Could you check a few things on this model? Use its own coordinates, in mm. Face numbers are marked on the shaded views. A direction names the side the tool comes from. Give positions to 0.01 mm unless a question says otherwise; leave off trailing zeros. Order: outer loops, then holes, each group sorted by start corner. A loop starts at its lowest first (then second) coordinate and runs counter-clockwise, first axis right, second up. Notation, with made-up numbers: (67.5, 76) -> (83.5, 76) arc R30 ccw to (83.5, 98) -> close; hole circle Ø4 at (-5, -13). An arc over 180 degrees is marked (long way). Write each question's results on one line, items separated by ' | '.
```python
from build123d import *

# Parameters (mm, degrees)
BOSS_EXTRU_1_DEPTH                                   = 15
ESQUISSE2_W                                          = 10
ESQUISSE2_H                                          = 25
ESQUISSE2_H_2                                        = 5
BOSS_EXTRU_2_DEPTH                                   = 6
D_GAGEMENT_M1_21_D                                   = 1.4
CHAMBRAGE_POUR_T_TE_CYLINDRIQUE_FENDUE_M_D           = 3.4
CHAMBRAGE_POUR_T_TE_CYLINDRIQUE_FENDUE_M_CBORE_D     = 6.5
CHAMBRAGE_POUR_T_TE_CYLINDRIQUE_FENDUE_M_CBORE_DEPTH = 2
CONG_1_R                                             = 10


with BuildPart() as part:
    # Esquisse1 → Boss.-Extru.1 (new body)
    with BuildSketch(Plane.XY):
        Polygon((0, 0), (-20, 0), (-20, 6), (-13, 6), (-13, 76), (13, 76), (13, 6), (20, 6), (20, 0), align=None)
    extrude(amount=BOSS_EXTRU_1_DEPTH)

    # Esquisse2 → Boss.-Extru.2 (add)
    with BuildSketch(Plane.XZ):
        with Locations((15, 27.5)):
            Rectangle(ESQUISSE2_W, ESQUISSE2_H)
        with Locations((-15, 17.5)):
            Rectangle(ESQUISSE2_W, ESQUISSE2_H_2)
    extrude(amount=-BOSS_EXTRU_2_DEPTH)

    # Dégagement M1.21 (through all)
    with Locations(Plane.XY.offset(15)):
        with Locations((0, 62), (0, 40)):
            Hole(D_GAGEMENT_M1_21_D / 2)

    # Chambrage pour tête cylindrique fendue M31 (through all)
    with Locations(Plane(origin=(0, 6, 0), x_dir=(1, 0, 0), z_dir=(0, 1, 0))):
        with Locations((-16.5, -5), (16.5, -5), (16.5, -35)):
            CounterBoreHole(CHAMBRAGE_POUR_T_TE_CYLINDRIQUE_FENDUE_M_D / 2, CHAMBRAGE_POUR_T_TE_CYLINDRIQUE_FENDUE_M_CBORE_D / 2, CHAMBRAGE_POUR_T_TE_CYLINDRIQUE_FENDUE_M_CBORE_DEPTH)

    # Congé1
    cong_1_edges = [part.edges().sort_by_distance(p)[0] for p in [
        (-13, 76, 7.5),
        (13, 76, 7.5),
    ]]
    fillet(cong_1_edges, radius=CONG_1_R)


solid = part.part
```
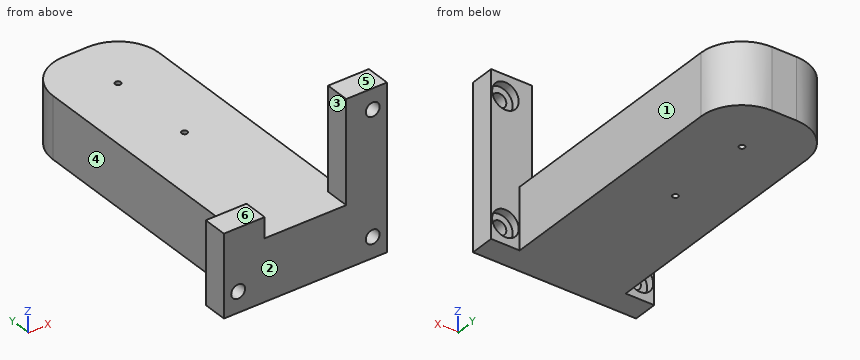
Q1. Suppose I cut it at B-B on x = 16.5. Please give me the cut outline in (y, z).
Here are the results:
outline: (0, 0) -> (6, 0) -> (6, 1.75) -> (4, 1.75) -> (4, 3.3) -> (0, 3.3) -> close; (0, 6.7) -> (4, 6.7) -> (4, 8.25) -> (6, 8.25) -> (6, 31.75) -> (4, 31.75) -> (4, 33.3) -> (0, 33.3) -> close; (0, 36.7) -> (4, 36.7) -> (4, 38.25) -> (6, 38.25) -> (6, 40) -> (0, 40) -> close
Q2. Suppose I cut it at A-A on z = 5. Please give me the cut outline in (x, y), and give its area (3 significant figures).
Here are the results:
outline: (-20, 0) -> (-18.2, 0) -> (-18.2, 4) -> (-19.75, 4) -> (-19.75, 6) -> (-20, 6) -> close; (-14.8, 0) -> (14.8, 0) -> (14.8, 4) -> (13.25, 4) -> (13.25, 6) -> (13, 6) -> (13, 66) arc R10 ccw to (3, 76) -> (-3, 76) arc R10 ccw to (-13, 66) -> (-13, 6) -> (-13.25, 6) -> (-13.25, 4) -> (-14.8, 4) -> close; (18.2, 0) -> (20, 0) -> (20, 6) -> (19.75, 6) -> (19.75, 4) -> (18.2, 4) -> close; hole circle Ø1.4 at (0, 40); hole circle Ø1.4 at (0, 62) | area: 1,960 mm²
Q3. Suppose I cut it at C-C on z = 35. Please give me the cut outline in (x, y).
Here are the results:
outline: (10, 0) -> (14.8, 0) -> (14.8, 4) -> (13.25, 4) -> (13.25, 6) -> (10, 6) -> close; (18.2, 0) -> (20, 0) -> (20, 6) -> (19.75, 6) -> (19.75, 4) -> (18.2, 4) -> close
Q4. I need wall thicknesses on line 1 along X through (y, z) = (1, 5); line 2 along Z through (x, y) = (16.5, 2.05); line 3 along Y through (x, z) = (0, 10.5). Which ranges of each line are inside material? Lowest first, please.
Here are the results:
line 1: x = -20 to -18.2, -14.8 to 14.8, 18.2 to 20 | line 2: z = 0 to 3.3, 6.7 to 33.3, 36.7 to 40 | line 3: y = 0 to 39.3, 40.7 to 61.3, 62.7 to 76
Q5. I'm going to push flat-ended pins straight in: pin 1 Ø8 at (y, z) = (17, 10.5) entering from +X; pin 2 Ø1.8 at (x, y) = (0, 62) entering from -Z; pin 3 Ø5 at (x, z) = (-17, 4.5) entering from +Y; pin 4 Ø10.5 at (x, z) = (-16.5, 5) entering from +Y. Where does each tip first touch, or does it pass through?
Here are the results:
pin 1: stops at x = 13 | pin 2: stops at z = 0 | pin 3: stops at y = 4 | pin 4: stops at y = 71.65
Q6. Suppose I cut it at D-D on x = -16. Please give me the cut outline in (y, z), and give its area (3 significant figures).
Here are the results:
outline: (0, 0) -> (6, 0) -> (6, 1.79) -> (4, 1.79) -> (4, 3.38) -> (0, 3.38) -> close; (0, 6.62) -> (4, 6.62) -> (4, 8.21) -> (6, 8.21) -> (6, 20) -> (0, 20) -> close | area: 94.2 mm²
Q7. For the marked faces 5 and 6, which set-ups out of +Z, -Z, +X, -X, +Y, -Y let a thin tool reach every point of the face, with its end or its side?
Here are the results:
face 5: +Z, +X, -X, +Y, -Y | face 6: +Z, -X, +Y, -Y
Q8. Thinking about a two-plate mould opening in X: for the marked faces 1, 2, 3 and 4, which applies, +X half, -X half, draft (parallel to the pull), parting line (faces both ways), or undercut?
Here are the results:
face 1: +X half | face 2: draft | face 3: undercut | face 4: -X half
